```python
from build123d import *

# Parameters (mm, degrees)
SKETCH2_R           = 23.5
BOSS_EXTRUDE1_DEPTH = 0.5
SKETCH3_R           = 0.75
CUT_EXTRUDE1_DEPTH  = 5


with BuildPart() as part:
    # Sketch1 → Revolve1 (revolve)
    with BuildSketch(Plane.XY, mode=Mode.PRIVATE) as revolve1_sk:
        Polygon((0, 0), (0, 4.850885244), (23.3, 4.850885244), (23.3, 5.500885244), (25.3, 5.500885244), (27.458615933, -0.499114756), (28.458615933, -0.499114756), (30, -5), (15, -5), (15, 0), align=None)
    revolve(revolve1_sk.sketch.rotate(Axis((0, 0, 0), (0, 1, 0)), 90), axis=Axis((0, 0, 0), (0, 1, 0)))

    # Sketch2 → Boss-Extrude1 (add)
    with BuildSketch(Plane(origin=(0, 4.850885244, 0), x_dir=(1, 0, 0), z_dir=(0, 1, 0))):
        Circle(SKETCH2_R)
    extrude(amount=BOSS_EXTRUDE1_DEPTH)

    # Sketch3 → Cut-Extrude1 (cut)
    with BuildSketch(Plane(origin=(0, 5.350885244, 0), x_dir=(1, 0, 0), z_dir=(0, 1, 0))):
        with Locations(Location((0, 17.004734632, 0), (0, 0, 270))):
            Circle(SKETCH3_R)
        with Locations(Location((0, -17.995265368, 0), (0, 0, 270))):
            Circle(SKETCH3_R)
    extrude(amount=-CUT_EXTRUDE1_DEPTH, mode=Mode.SUBTRACT)


solid = part.part
```
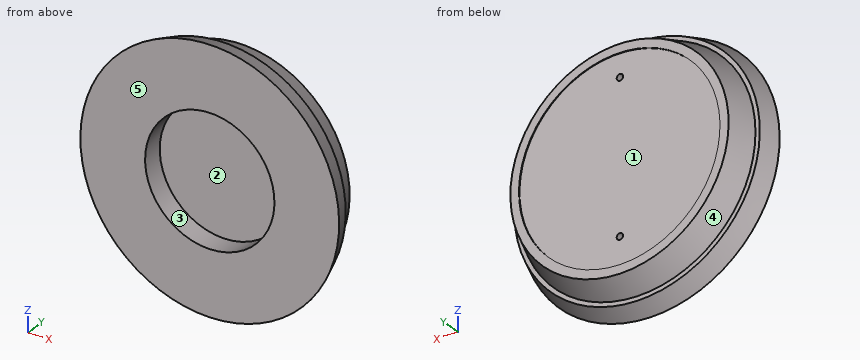
The listing builds one solid part. Answer for the finished solid, in the listing's coordinates (mm). Face numbers are marked on the shaded views. A direction names the side the tool comes from. Give positions to 0.01 mm unless a question says otherwise; leave off trailing zeros. Loops run counter-clockwise (first coordinate to the right, second up) from the corner with the lowest first, then second, coordinate; pieces in that order, holes last. Notation, with made-up numbers: (-5, 2) - (32, 2) arc R6 cw to (32, 7) - close; hole circle Ø11 at (50, -28). An arc over 180 degrees is marked (long way). Answer as CSV lines item,"result". Start each with the question number.
Item 1: A cutting plane is placed at D-D on y = 3.5. Determine the outline of the cut face in (x, z), then the cut area to 3 significant figures.
Item 2: A cutting plane is placed at C-C on y = -2.5. Determine the outline of the cut face in (x, z).
Item 3: A cutting plane is placed at B-B on x = 0. Determine the outline of the cut face in (y, z).
Item 4: Find the intervals of material crossed by line 1 (X direction, y = 5.45, z = 0); line 2 (Y direction, x = -11.5, z = 14); line 3 (Y direction, x = -20.5, z = -18), in increasing order. Write a range as from..to.
Item 5: Each of these flat-tipped pins is pushed along its axis until it touches: pin 1 (5 mm diameter, centred on y = 4, z = -23.5, fed in from -X); pin 2 (5 mm diameter, centred on x = -17, y = -0.5, fed in from -Z); pin 3 (8 mm diameter, centred on x = 1, z = 6.5, fed in from -Y). Where does it stop, or does it pass through?
Item 6: For the marked faces 1 and 2, determine the directions among +Z, -Z, +X, -X, +Y, -Y from which every point of the face is accessible in a straight line to the end or side of a thin tool.
Item 7: The mould has two halves that part along Z. Classify the marked faces 3, 4 and 5: +Z half, -Z half, draft (parallel to the pull), parting line (faces both ways), or undercut.
Item 8: A cutting plane is placed at A-A on z = 0. Determine the outline of the cut face in (x, y).
Found:
1,outline,"circle Ø52.04 at (0, 0); hole circle Ø1.5 at (0, -17); hole circle Ø1.5 at (0, 18)"
1,area,"2,120 mm^2"
2,outline,"circle Ø58.29 at (0, 0); hole circle Ø30 at (0, 0)"
3,outline,"(-5, -30) - (-0.5, -28.46) - (-0.5, -27.46) - (5.5, -25.3) - (5.5, -23.3) - (5.35, -23.3) - (5.35, -17.75) - (0.35, -17.75) - (0.35, -16.25) - (5.35, -16.25) - (5.35, 17.25) - (0.35, 17.25) - (0.35, 18.75) - (5.35, 18.75) - (5.35, 23.3) - (5.5, 23.3) - (5.5, 25.3) - (-0.5, 27.46) - (-0.5, 28.46) - (-5, 30) - (-5, 15) - (0, 15) - (0, -15) - (-5, -15) - close"
4,line 1,"x = -25.32..-23.3, 23.3..25.32"
4,line 2,"y = -5..5.35"
4,line 3,"y = -5..-0.01"
5,pin 1,"stops at x = -15.38"
5,pin 2,"stops at z = -24.79"
5,pin 3,"stops at y = 0"
6,face 1,"+Y"
6,face 2,"-Y"
7,face 3,"undercut"
7,face 4,"parting line"
7,face 5,"draft"
8,outline,"(-30, -5) - (-15, -5) - (-15, 0) - (15, 0) - (15, -5) - (30, -5) - (28.46, -0.5) - (27.46, -0.5) - (25.3, 5.5) - (23.3, 5.5) - (23.3, 5.35) - (-23.3, 5.35) - (-23.3, 5.5) - (-25.3, 5.5) - (-27.46, -0.5) - (-28.46, -0.5) - close"
